Source: CAD feature listing. Evaluate the final solid. Frame: model axes, mm. A direction names the side the tool comes from. Give positions to 0.01 mm unless a question says otherwise; leave off trailing zeros. Order: outer loops, then holes, each group sorted by start corner. A loop starts at its lowest first (then second) coordinate and runs counter-clockwise, first axis right, second up.
1) Draft query along X for faces 1 (the face through (7, 0.5, 1)), 2 (the face through (4.662, -1.549, 0.986)), 3 (the face through (0.73, -1.94, 0.99)). Return one class per face: released by +X, released by -X, zero draft, split by the parting line, or undercut.
2) Section A-A, the plane y = -50.5. Return loops of the section in (x, z), plus the area to 3 significant figures.
3) Section B-B, the plane z = 0.85. Return loops of the section in (x, y).
4) First-contact query: P1, Ø0.6, axis at x = 4.5, z = 0.5, coming from the -Y side; P2, Ø1, axis at y = -35.5, z = 0.5, coming from the -X side. Flat tips, straight axial feed; report the tip coordinate or a pass-through.
5) Material intervals for line 1 (Y direction, x = 3.5, z = 2.1); line 2 (X direction, y = -48, z = 0.35); line 3 (Y direction, x = 3.25, z = 2.5), sorted ascending.
6) Access query for faces 4 (the face through (5, -4.5, 1)), 5 (the face through (8.626, -67.513, 0.986)). Directions: +Z, -Z, +X, -X, +Y, -Y. A direction counts if a zero-diameter tool reaches every point of the face in a straight line with its end or side. Return the directions, or none.
```python
from build123d import *

# Parameters (mm, degrees)
SKETCH1_R           = 1.5
BOSS_EXTRUDE1_DEPTH = 3
FILLET1_R           = 1


with BuildPart() as part:
    # Sketch1 → Boss-Extrude1 (new body)
    with BuildSketch(Plane.XY):
        with BuildLine():
            Line((3.231167374, -4.499889348), (6.321167374, -4.499889348))
            Line((6.321167374, -4.499889348), (6.321167374, -68.999889348))
            ThreePointArc((6.321167374, -68.999889348), (8.821167374, -71.499889348), (11.321167374, -68.999889348))
            Line((11.321167374, -68.999889348), (11.321167374, 0.500110652))
            Line((11.321167374, 0.500110652), (3.231167374, 0.500110652))
            ThreePointArc((3.231167374, 0.500110652), (0.731167374, -1.999889348), (3.231167374, -4.499889348))
        make_face()
        with Locations((3.231167374, -1.999889348)):
            Circle(SKETCH1_R, mode=Mode.SUBTRACT)
        with Locations((8.821167374, -68.999889348)):
            Circle(SKETCH1_R, mode=Mode.SUBTRACT)
    extrude(amount=BOSS_EXTRUDE1_DEPTH)

    # Fillet1
    # the kernel refuses this fillet: 1 mm, written as the material it takes off along each edge
    with BuildSketch(Plane(origin=(8.821167374, -68.999889348, 3), x_dir=(1, 0, 0), z_dir=(0, -1, 0))) as fillet1_piece_1:
        with BuildLine():
            CenterArc((1.5 + FILLET1_R, -FILLET1_R), FILLET1_R, 90, 90)
            Line((1.5 + FILLET1_R, 0), (1.5, 0))
            Line((1.5, 0), (1.5, -FILLET1_R))
        make_face()
    revolve(axis=Axis((8.821167374, -68.999889348, 3), (0, 0, 1)), mode=Mode.SUBTRACT)
    with BuildSketch(Plane(origin=(3.231167374, -1.999889348, 3), x_dir=(1, 0, 0), z_dir=(0, -1, 0))) as fillet1_piece_2:
        with BuildLine():
            CenterArc((1.5 + FILLET1_R, -FILLET1_R), FILLET1_R, 90, 90)
            Line((1.5 + FILLET1_R, 0), (1.5, 0))
            Line((1.5, 0), (1.5, -FILLET1_R))
        make_face()
    revolve(axis=Axis((3.231167374, -1.999889348, 3), (0, 0, 1)), mode=Mode.SUBTRACT)
    with BuildSketch(Plane(origin=(13.821167374, 0.500110652, 3), x_dir=(0, 0, -1), z_dir=(-1, 0, 0))) as fillet1_piece_3:
        with BuildLine():
            CenterArc((FILLET1_R, FILLET1_R), FILLET1_R, 180, 90)
            Line((0, FILLET1_R), (0, 0))
            Line((0, 0), (FILLET1_R, 0))
        make_face()
    extrude(amount=10.59, mode=Mode.SUBTRACT)
    with BuildSketch(Plane(origin=(11.321167374, -68.999889348, 3), x_dir=(0, 0, -1), z_dir=(0, 1, 0))) as fillet1_piece_4:
        with BuildLine():
            CenterArc((FILLET1_R, FILLET1_R), FILLET1_R, 180, 90)
            Line((0, FILLET1_R), (0, 0))
            Line((0, 0), (FILLET1_R, 0))
        make_face()
    extrude(amount=72, mode=Mode.SUBTRACT)
    with BuildSketch(Plane(origin=(8.821167374, -68.999889348, 3), x_dir=(-1, 0, 0), z_dir=(0, 1, 0))) as fillet1_piece_5:
        with BuildLine():
            CenterArc((2.5 - FILLET1_R, -FILLET1_R), FILLET1_R, 0, 90)
            Line((2.5 - FILLET1_R, 0), (2.5, 0))
            Line((2.5, 0), (2.5, -FILLET1_R))
        make_face()
    revolve(axis=Axis((8.821167374, -68.999889348, 3), (0, 0, 1)), revolution_arc=180, mode=Mode.SUBTRACT)
    with BuildSketch(Plane(origin=(6.321167374, -4.499889348, 3), x_dir=(0, 0, -1), z_dir=(0, -1, 0))) as fillet1_piece_6:
        with BuildLine():
            CenterArc((FILLET1_R, FILLET1_R), FILLET1_R, 180, 90)
            Line((0, FILLET1_R), (0, 0))
            Line((0, 0), (FILLET1_R, 0))
        make_face()
    extrude(amount=64.5, mode=Mode.SUBTRACT)
    with BuildSketch(Plane(origin=(3.231167374, -4.499889348, 3), x_dir=(0, 0, -1), z_dir=(1, 0, 0))) as fillet1_piece_7:
        with BuildLine():
            CenterArc((FILLET1_R, FILLET1_R), FILLET1_R, 180, 90)
            Line((0, FILLET1_R), (0, 0))
            Line((0, 0), (FILLET1_R, 0))
        make_face()
    extrude(amount=3.09, mode=Mode.SUBTRACT)
    with BuildSketch(Plane(origin=(3.231167374, -1.999889348, 3), x_dir=(0, 1, 0), z_dir=(1, 0, 0))) as fillet1_piece_8:
        with BuildLine():
            CenterArc((2.5 - FILLET1_R, -FILLET1_R), FILLET1_R, 0, 90)
            Line((2.5 - FILLET1_R, 0), (2.5, 0))
            Line((2.5, 0), (2.5, -FILLET1_R))
        make_face()
    revolve(axis=Axis((3.231167374, -1.999889348, 3), (0, 0, 1)), revolution_arc=180, mode=Mode.SUBTRACT)
    with BuildSketch(Plane(origin=(3.231167374, -4.499889348, 3), x_dir=(0, 0, -1), z_dir=(1, 0, 0))) as fillet1_piece_9a_section:
        with BuildLine():
            CenterArc((FILLET1_R, FILLET1_R), FILLET1_R, 180, 90)
            Line((0, FILLET1_R), (0, 0))
            Line((0, 0), (FILLET1_R, 0))
        make_face()
    fillet1_piece_9a = extrude(amount=5.59, mode=Mode.PRIVATE)
    fillet1_piece_9a = split(fillet1_piece_9a, bisect_by=Plane(origin=(6.321167374, -4.273494233, 2.773604886), z_dir=(1, 0, 0)), keep=Keep.TOP, mode=Mode.PRIVATE)
    with BuildSketch(Plane(origin=(6.321167374, -1.999889348, 3), x_dir=(0, 0, -1), z_dir=(0, -1, 0))) as fillet1_piece_9b_section:
        with BuildLine():
            CenterArc((FILLET1_R, FILLET1_R), FILLET1_R, 180, 90)
            Line((0, FILLET1_R), (0, 0))
            Line((0, 0), (FILLET1_R, 0))
        make_face()
    fillet1_piece_9b = extrude(amount=67, mode=Mode.PRIVATE)
    fillet1_piece_9b = split(fillet1_piece_9b, bisect_by=Plane(origin=(6.547562488, -4.499889348, 2.773604886), z_dir=(0, 1, 0)), keep=Keep.TOP, mode=Mode.PRIVATE)
    fillet1_piece_9 = fillet1_piece_9a & fillet1_piece_9b
    add(fillet1_piece_9, mode=Mode.SUBTRACT)


solid = part.part
```
From the geometry:
1. face 1: zero draft
1. face 2: undercut
1. face 3: released by -X
2. outline: (6.32, 0) - (11.32, 0) - (11.32, 2) arc R1 ccw to (10.32, 3) - (7.32, 3) arc R1 ccw to (6.32, 2) - close
2. area: 14.6 mm2
3. outline: (3.23, -4.5) - (6.32, -4.5) - (6.32, -69) arc R2.5 ccw to (11.32, -69) - (11.32, 0.5) - (3.23, 0.5) arc R2.5 ccw to start; hole circle Ø3 at (3.23, -2); hole circle Ø3 at (8.82, -69)
4. P1: stops at y = -4.5
4. P2: stops at x = 6.32
5. line 1: y = -4.49 to -3.48, -0.52 to 0.5
5. line 2: x = 6.32 to 11.32
5. line 3: y = -4.37 to -3.63, -0.37 to 0.37
6. face 4: +Z, -Z, -X, -Y
6. face 5: +Z, -Z
